Check sheet for the modelled part. Datum: model origin and axes. Units: mm. A direction names the side the tool comes from. Round coordinates to 2 decimals unless told otherwise and drop trailing zeros. Write each loop counter-clockwise with the first axis right and the second up, starting at its lowest first coordinate (ties: lowest second). Pieces come first, ordered by that corner, then holes. Notation, with made-up numbers: (69.25, 31.25) - (118.25, 31.25) arc R22 ccw to (118.25, 63.25) - close; hole circle Ø8 at (13, -17.75). An arc over 180 degrees is marked (long way). Answer as a JSON object with one key per item and string values. Group by question number.
Item 1: Sectioned sample at B-B on y = 16. Record the boundary of the cut face in (x, z), plus the area to 3 significant figures.
Item 2: Gauge pin test, flat ends, axial feed: P1, Ø7.5, axis at y = 74, z = 37, coming from the +X side; P2, Ø4, axis at x = 12, z = -172, coming from the +Y side; P3, Ø10.5, axis at x = 11.55, z = 104.55, coming from the -Y side (3 decimals). Record the tip position at first contact, or that the pin passes through.
Item 3: Thickness scan on line 1 (X direction, y = 17, z = 104); line 2 (Z direction, x = 11.55, y = 20.5); line 3 (Z direction, x = 8, y = 19.5). Record the ranges inside material, lowest first.
Item 4: Set-up check for faces 1 (the flat face through (4.05, 5, 4)), 2 (the flat face through (9.39, 37.96, -285.16)), 3 (the flat face through (12, 70, 4)): record each of +Z, -Z, +X, -X, +Y, -Y from which the full face is reachable in a straight line by a thin tool's end or side.
Item 5: Sectioned sample at C-C on y = 41.5. Record the boundary of the cut face in (x, z), plus the area to 3 significant figures.
```python
from build123d import *

# Parameters (mm, degrees)
BOSS_EXTRUDE1_DEPTH            = 294.550000053
FILLET1_R                      = 1.5875
CUT_EXTRUDE1_DEPTH             = 306.043611732
CUT_EXTRUDE1_DEPTH_BACK        = 306.043611732
F_7_9_7_9_DIAMETER_HOLE2_D     = 7.9
F_7_9_7_9_DIAMETER_HOLE2_DEPTH = 15
F_7_9_7_9_DIAMETER_HOLE2_TIP   = 2.373399445


with BuildPart() as part:
    # Sketch1 → Boss-Extrude1 (new, symmetric)
    with BuildSketch(Plane.XY):
        Polygon((0, 77.000000178), (0, 0), (4.050000028, 0), (4.050000028, 9.525), (19.05, 9.525), (19.05, 70.000000208), (4.050000028, 70.000000208), (4.050000028, 77.000000178), align=None)
    extrude(amount=BOSS_EXTRUDE1_DEPTH, both=True)

    # Fillet1
    fillet1_edges = [part.edges().sort_by_distance(p)[0] for p in [
        (0, 0, 0),
        (0, 77.000000178, 0),
    ]]
    fillet(fillet1_edges, radius=FILLET1_R)

    # Sketch2 → Cut-Extrude1 (cut, two sides: drawn at the far end of the back side and taken through both)
    with BuildSketch(Plane(origin=(0, 77.000000178, 0), x_dir=(1, 0, 0), z_dir=(0, 1, 0)).offset(-CUT_EXTRUDE1_DEPTH_BACK)):
        Polygon((0, 294.550000053), (19.05, 275.500000053), (19.05, 294.550000053), align=None)
        Polygon((19.05, -275.500000053), (19.05, -294.550000053), (0, -294.550000053), align=None)
    extrude(amount=CUT_EXTRUDE1_DEPTH + CUT_EXTRUDE1_DEPTH_BACK, mode=Mode.SUBTRACT)

    # Ø7.9 (7.9) Diameter Hole2
    with Locations(Plane.XZ.offset(-9.525)):
        with Locations((11.550000014, -104.550000053), (11.550000014, 104.550000053)):
            Hole(F_7_9_7_9_DIAMETER_HOLE2_D / 2, depth=F_7_9_7_9_DIAMETER_HOLE2_DEPTH)
            with Locations((0, 0, -(F_7_9_7_9_DIAMETER_HOLE2_DEPTH + F_7_9_7_9_DIAMETER_HOLE2_TIP / 2))):  # 118° drill point
                Cone(0, F_7_9_7_9_DIAMETER_HOLE2_D / 2, F_7_9_7_9_DIAMETER_HOLE2_TIP, mode=Mode.SUBTRACT)


solid = part.part
```
Completed:
{
 "1": {"outline": "(0, -294.55) - (19.05, -275.5) - (19.05, 275.5) - (0, 294.55) - close; hole circle Ø7.9 at (11.55, -104.55); hole circle Ø7.9 at (11.55, 104.55)", "area": "10,800 mm²"},
 "2": {"P1": "x = 4.05", "P2": "y = 70", "P3": "y = 9.525"},
 "3": {"line 1": "0 to 7.64, 15.46 to 19.05", "line 2": "-283 to -108.5, -100.6 to 100.6, 108.5 to 283", "line 3": "-286.55 to -106.28, -102.82 to 102.82, 106.28 to 286.55"},
 "4": {"face 1": "+Z, -Z, +X, -Y", "face 2": "-Z, +X, +Y, -Y", "face 3": "+Z, -Z, +X, +Y"},
 "5": {"outline": "(0, -294.55) - (19.05, -275.5) - (19.05, 275.5) - (0, 294.55) - close", "area": "10,900 mm²"}
}
